```python
from build123d import *

# Parameters (mm, degrees)
F0_R     = 23.8125
F1_DEPTH = 19.05
F0_R_2   = 12.7
F2_DEPTH = 6.35
F3_SIZE  = 0.508
F4_R     = 2.54
F5_DEPTH = 25.4
F6_R     = 3.175


with BuildPart() as f1:
    # F0 (on Right) → F1 (new body)
    with BuildSketch(Plane.YZ):
        with BuildLine():
            Line((50.8, -152.4), (37.971048, 3.132016))
            ThreePointArc((37.971048, 3.132016), (0, 38.1), (-37.971048, 3.132016))
            Line((-37.971048, 3.132016), (-50.8, -152.4))
            Line((-50.8, -152.4), (50.8, -152.4))
        make_face()
        Circle(F0_R, mode=Mode.SUBTRACT)
    extrude(amount=F1_DEPTH)

    # F0 (on Right) → F2 (join)
    with BuildSketch(Plane.YZ):
        Circle(F0_R)
        Circle(F0_R_2, mode=Mode.SUBTRACT)
    extrude(amount=F2_DEPTH)

    # F3
    f3_edges = [f1.edges().sort_by_distance(p)[0] for p in [
        (6.35, -12.7, 0),
        (19.05, -23.8125, 0),
        (0, -12.7, 0),
    ]]
    chamfer(f3_edges, length=F3_SIZE)

    # F4 (on face) → F5 (cut)
    with BuildSketch(Plane(origin=(0, 0, -152.4), x_dir=(1, 0, 0), z_dir=(0, 0, -1))):
        with Locations((9.525, 25.4)):
            Circle(F4_R)
        with Locations((9.525, -25.4)):
            Circle(F4_R)
    extrude(amount=-F5_DEPTH, mode=Mode.SUBTRACT)

    # F6
    f6_edges = [f1.edges().sort_by_distance(p)[0] for p in [
        (19.05, -44.385524, -74.633992),
        (0, -44.385524, -74.633992),
    ]]
    fillet(f6_edges, radius=F6_R)


solid = f1.part
```
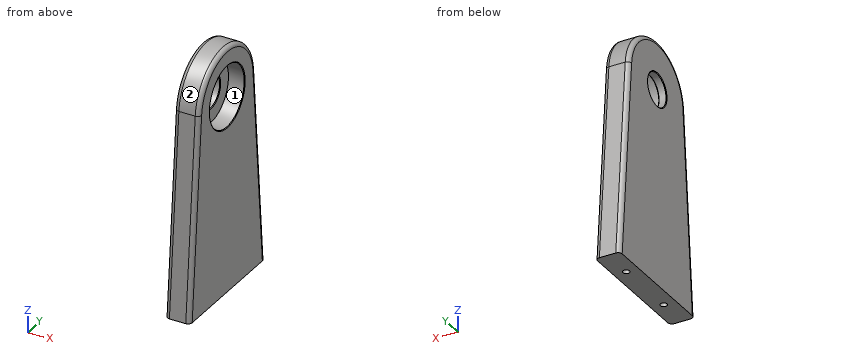
Can you work these out from the model? Positions are in its coordinate system, mm. Face numbers are marked on the shaded views. A direction names the side the tool comes from. Coordinates: 2 decimals unless noted, no trailing zeros. Order: outer loops, then holes, each group sorted by start corner. A loop starts at its lowest first (then second) coordinate and runs counter-clockwise, first axis right, second up.
1. If we section it at B-B (x = 9): Please give me the cut outline in (y, z) (1 decimal), then the cut area to 3 significant figures.
2. I'm going to push flat-ended pins straight in: pin 1 (6.5 mm diameter, centred on x = 9.525, y = 25.4, fed in from +Z); pin 2 (5 mm diameter, centred on x = 11.5, y = 3.5, fed in from +Z); pin 3 (2 mm diameter, centred on x = 7.5, z = -96.5, fed in from -Y); pin 4 (4 mm diameter, centred on x = 9.5, y = -26.5, fed in from -Z). Where does each tip first touch, or does it pass through?
3. For the marked faces 1 and 2, which set-ups out of +Z, -Z, +X, -X, +Y, -Y let a thin tool reach every point of the face, with its end or its side?
4. If we section it at C-C (z = -130): Give the number of separate pieces and of enclosed holes in the cut face, then the cut area to 3 significant figures.
5. I need wall thicknesses on line 1 (X direction, y = 25, z = -144); line 2 (X direction, y = -25.4, z = -140) (3 decimals); line 3 (Y direction, x = 11, z = -128). Which ranges of each line are inside material? Lowest first, please.
Entries:
1. outline: (-50.8, -152.4) - (-27.9, -152.4) - (-27.9, -127) - (-22.9, -127) - (-22.9, -152.4) - (22.9, -152.4) - (22.9, -127) - (27.9, -127) - (27.9, -152.4) - (50.8, -152.4) - (38, 3.1) arc R38.1 ccw to (-38, 3.1) - close; hole circle Ø47.6 at (0, 0)
1. area: 13,800 mm2
2. pin 1: stops at z = 31
2. pin 2: stops at z = 38.09
2. pin 3: stops at y = -46.27
2. pin 4: stops at z = -152.4
3. face 1: +X
3. face 2: +Z, +X, -X
4. separate pieces: 1
4. enclosed holes: 2
4. area: 1,820 mm2
5. line 1: x = 0 to 7.02, 12.03 to 19.05
5. line 2: x = 0 to 6.985, 12.065 to 19.05
5. line 3: y = -48.79 to -27.47, -23.33 to 23.33, 27.47 to 48.79
